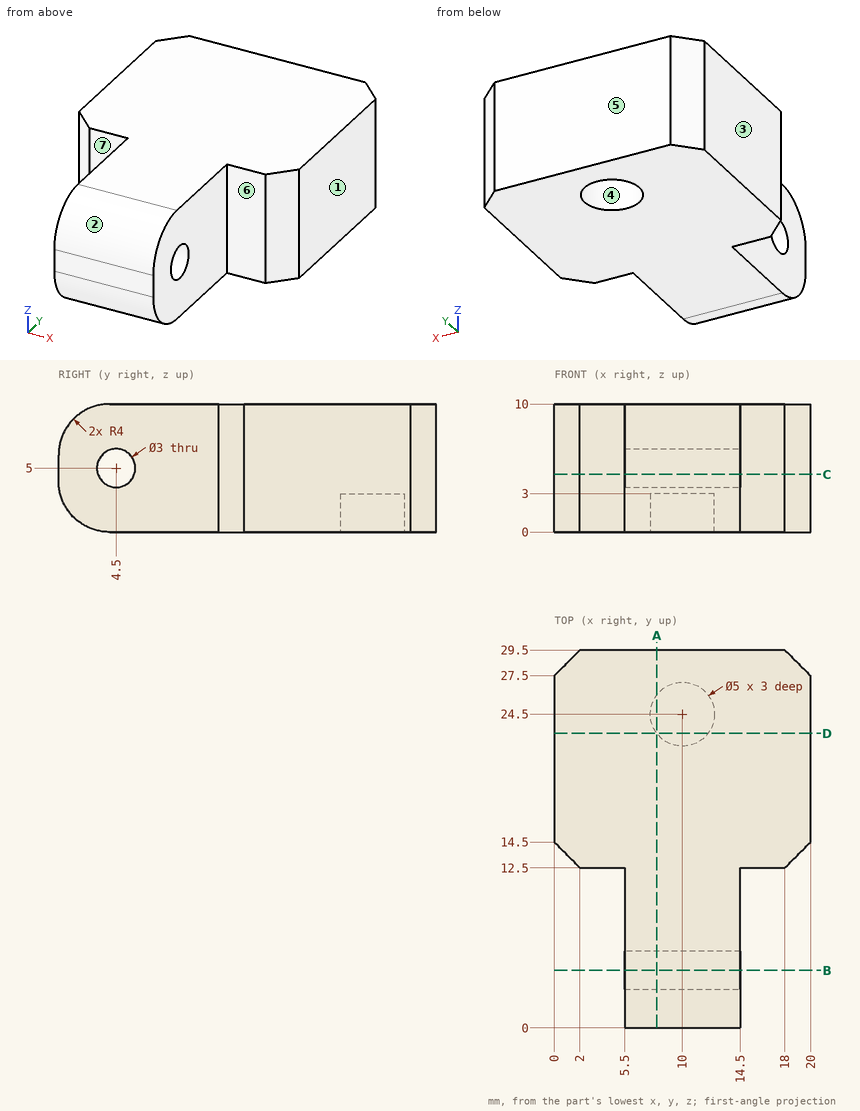
Input: dimensioned drawing with shaded views. Units: mm. Origin: part minimum x, y, z. A direction names the side the tool comes from. Coordinates: 2 decimals unless noted, no trailing zeros. Write each loop counter-clockwise with the first axis right and the second up, starting at its lowest first coordinate (ties: lowest second). Pieces come first, ordered by that corner, then holes. Notation, with made-up numbers: M -37.5,28.5 L -27.5,28.5 A16 cw -27.5,39.5 Z; hole C -14.5,-13.5 d4. An arc over 180 degrees is marked long. Use a Markdown table: item, result.
1) Ray query, L1, parallel to X at y = 24.5, z = 1.25; L2, parallel to Z at x = 11.25, y = 4.5; L3, parallel to X at y = 12.25, z = 3.75. Return the intervals inside material, ascending.
Conclusion:
| item | result |
|---|---|
| L1 | x = 0 to 7.5, 12.5 to 20 |
| L2 | z = 0 to 3.5, 6.5 to 10 |
| L3 | x = 5.5 to 14.5 |
2) Section C-C, the plane z = 4.5. Output: boundary loops of the cut face in (x, y), then the cut area to 3 significant figures.
Conclusion:
| item | result |
|---|---|
| outline | M 0,14.5 L 2,12.5 L 5.5,12.5 L 5.5,5.91 L 14.5,5.91 L 14.5,12.5 L 18,12.5 L 20,14.5 L 20,27.5 L 18,29.5 L 2,29.5 L 0,27.5 Z; M 5.5,0 L 14.5,0 L 14.5,3.09 L 5.5,3.09 Z |
| area | 419 mm^2 |
3) Section B-B, the plane y = 4.5. Output: boundary loops of the cut face in (x, z), then the cut area to 3 significant figures.
Conclusion:
| item | result |
|---|---|
| outline | M 5.5,0 L 14.5,0 L 14.5,3.5 L 5.5,3.5 Z; M 5.5,6.5 L 14.5,6.5 L 14.5,10 L 5.5,10 Z |
| area | 63.0 mm^2 |
4) Section D-D, the plane y = 23. Output: boundary loops of the cut face in (x, z), then the cut area to 3 significant figures.
Conclusion:
| item | result |
|---|---|
| outline | M 0,0 L 8,0 L 8,3 L 12,3 L 12,0 L 20,0 L 20,10 L 0,10 Z |
| area | 188 mm^2 |
5) Section A-A, the plane x = 8. Output: boundary loops of the cut face in (y, z), then the cut area to 3 significant figures.
Conclusion:
| item | result |
|---|---|
| outline | M 0,4 A4 ccw 4,0 L 23,0 L 23,3 L 26,3 L 26,0 L 29.5,0 L 29.5,10 L 4,10 A4 ccw 0,6 Z; hole C 4.5,5 d3 |
| area | 272 mm^2 |
6) Mould query, pull axis X, two halves, no side actions, for the marked faces 1, 2, 3 and 4. Classes: pulls with the +X half, pulls with the -X half, needs draft (parallel to the pull), parting line crosses it, or undercut.
Conclusion:
| item | result |
|---|---|
| face 1 | pulls with the +X half |
| face 2 | needs draft |
| face 3 | pulls with the -X half |
| face 4 | undercut |
7) Reachability of the marked faces 5, 6 and 7 from +Z, -Z, +X, -X, +Y, -Y: full face, straight path, thin tool, end or side. Return the list, or none.
Conclusion:
| item | result |
|---|---|
| face 5 | +Z, -Z, +X, -X, +Y |
| face 6 | +Z, -Z, +X, -Y |
| face 7 | +Z, -Z, -X, -Y |
8) First-contact query: pin 1 Ø2 at (y, z) = (13, 6) entering from +X; pin 2 Ø3 at (y, z) = (3.5, 2) entering from +X; pin 3 Ø1.5 at (x, y) = (9.5, 25.5) entering from -Z. Flat tips, straight axial feed; report the tip coordinate or a pass-through.
Conclusion:
| item | result |
|---|---|
| pin 1 | stops at x = 19.5 |
| pin 2 | stops at x = 14.5 |
| pin 3 | stops at z = 3 |
